```python
from build123d import *

# Parameters (mm, degrees)
IZIM1_R                     = 2.5
Y_KSEKLIK_EKSTR_ZYON1_DEPTH = 25
IZIM2_W                     = 20
IZIM2_H                     = 40
KES_EKSTR_ZYON1_DEPTH       = 47
RADYUS1_R                   = 5
IZIM3_R                     = 2.5
KES_EKSTR_ZYON3_DEPTH       = 47


with BuildPart() as part:
    # Çizim1 → Yükseklik-Ekstrüzyon1 (new body)
    with BuildSketch(Plane.XY):
        with BuildLine():
            Line((-30.949719985, 7.301527432), (-30.949719985, -22.698472568))
            Line((-30.949719985, -22.698472568), (-0.949719985, -22.698472568))
            Line((-0.949719985, -22.698472568), (-0.949719985, 7.301527432))
            ThreePointArc((-0.949719985, 7.301527432), (-15.949719985, 22.301527432), (-30.949719985, 7.301527432))
        make_face()
        with Locations((-15.949719985, 7.301527432)):
            Circle(IZIM1_R, mode=Mode.SUBTRACT)
    extrude(amount=Y_KSEKLIK_EKSTR_ZYON1_DEPTH)

    # Çizim2 → Kes-Ekstrüzyon1 (cut)
    with BuildSketch(Plane(origin=(0, 0, 0), x_dir=(0, 0, -1), z_dir=(1, 0, 0))):
        with Locations((-10, 2.301527432)):
            Rectangle(IZIM2_W, IZIM2_H)
    extrude(amount=-KES_EKSTR_ZYON1_DEPTH, mode=Mode.SUBTRACT)

    # Radyus1
    radyus1_edges = [part.edges().sort_by_distance(p)[0] for p in [
        (-30.949719985, -20.198472568, 0),
        (-0.949719985, -20.198472568, 0),
    ]]
    fillet(radyus1_edges, radius=RADYUS1_R)

    # Çizim3 → Kes-Ekstrüzyon3 (cut)
    with BuildSketch(Plane(origin=(0, 0, 0), x_dir=(1, 0, 0), z_dir=(0, 1, 0))):
        with Locations(Location((-23.449719985, -15, 0), (0, 0, 270))):
            Circle(IZIM3_R)
        with Locations(Location((-8.449719985, -15, 0), (0, 0, 270))):
            Circle(IZIM3_R)
    extrude(amount=-KES_EKSTR_ZYON3_DEPTH, mode=Mode.SUBTRACT)


solid = part.part
```
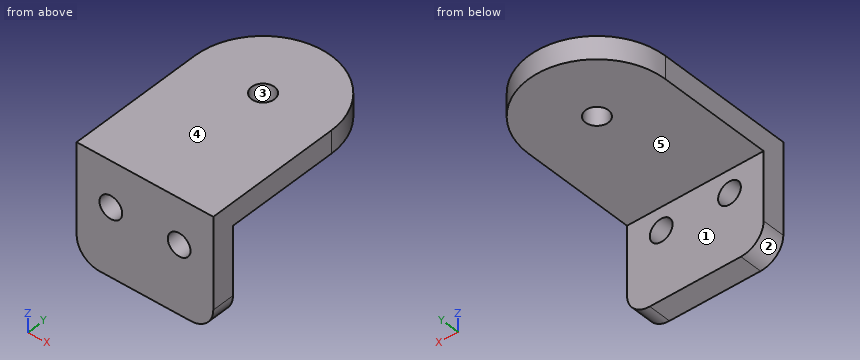
Work out the finished part from the listing and answer in its coordinate system (mm). Face numbers are marked on the shaded views. A direction names the side the tool comes from. Coordinates: 2 decimals unless noted, no trailing zeros. Loops run counter-clockwise (first coordinate to the right, second up) from the corner with the lowest first, then second, coordinate; pieces in that order, holes last. Notation, with made-up numbers: (81, 13) -> (88, 13) arc R24 ccw to (88, 38) -> close; hole circle Ø4 at (61.5, 5). An arc over 180 degrees is marked (long way). Answer as CSV lines item,"result".
Q1. The part is cut by section B-B on x = -24. Write down the section's boundary in (y, z), and give its area (3 significant figures).
Findings:
outline,"(-22.7, 0) -> (-17.7, 0) -> (-17.7, 12.56) -> (-22.7, 12.56) -> close; (-22.7, 17.44) -> (-17.7, 17.44) -> (-17.7, 20) -> (19.96, 20) -> (19.96, 25) -> (-22.7, 25) -> close"
area,"289 mm²"
Q2. The part is cut by section A-A on z = 15. Write down the section's boundary in (x, y).
Findings:
outline,"(-30.95, -22.7) -> (-25.95, -22.7) -> (-25.95, -17.7) -> (-30.95, -17.7) -> close; (-20.95, -22.7) -> (-10.95, -22.7) -> (-10.95, -17.7) -> (-20.95, -17.7) -> close; (-5.95, -22.7) -> (-0.95, -22.7) -> (-0.95, -17.7) -> (-5.95, -17.7) -> close"
Q3. The part is cut by section C-C on y = 8. Write down the section's boundary in (x, z), and give its area (3 significant figures).
Findings:
outline,"(-30.93, 20) -> (-18.35, 20) -> (-18.35, 25) -> (-30.93, 25) -> close; (-13.55, 20) -> (-0.97, 20) -> (-0.97, 25) -> (-13.55, 25) -> close"
area,"126 mm²"
Q4. Find the intervals of material crossed by probe 1 along X at (y, z) = (-18.85, 15); probe 2 along X at (y, z) = (-19.5, 16.5); probe 3 along Z at (x, y) = (-15, 11.5), in increasing order.
Findings:
probe 1,"x = -30.95 to -25.95, -20.95 to -10.95, -5.95 to -0.95"
probe 2,"x = -30.95 to -25.45, -21.45 to -10.45, -6.45 to -0.95"
probe 3,"z = 20 to 25"
Q5. Each of these flat-tipped pins is pushed along its axis until it touches: pin 1 (6 mm diameter, centred on x = -8.45, z = 15, fed in from +Y); pin 2 (5 mm diameter, centred on x = -13, y = -4, fed in from -Z). Where does it stop, or does it pass through?
Findings:
pin 1,"stops at y = -17.7"
pin 2,"stops at z = 20"
Q6. For a pull along Y with two mould halves and no side action, classify the marked faces 1, 2 and 3 as +Y half, -Y half, draft (parallel to the pull), parting line (faces both ways), or undercut.
Findings:
face 1,"+Y half"
face 2,"draft"
face 3,"undercut"
Q7. The part is cut by section D-D on z = 20.5. Write down the section's boundary in (x, y).
Findings:
outline,"(-30.95, -22.7) -> (-0.95, -22.7) -> (-0.95, 7.3) arc R15 ccw to (-30.95, 7.3) -> close; hole circle Ø5 at (-15.95, 7.3)"
Q8. A tool of negligible diameter and unlimited length cuts with its end or side. For the marked faces 4 and 5, from which of +Z, -Z, +X, -X, +Y, -Y can it reach the whole face along a straight path? Write none if from no direction.
Findings:
face 4,"+Z, +X, -X, +Y, -Y"
face 5,"-Z, +X, -X, +Y"
